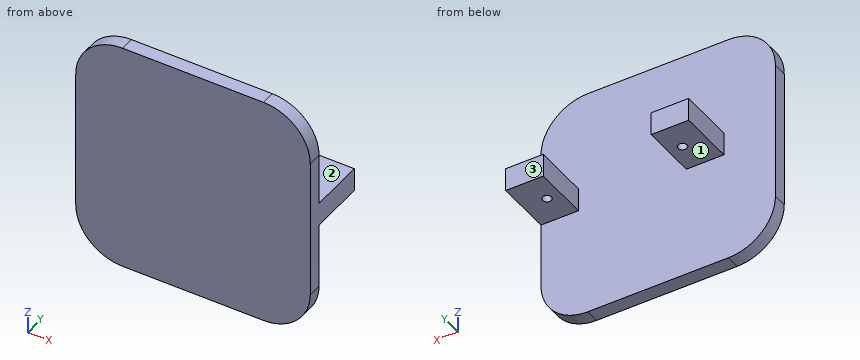
```python
from build123d import *

# Parameters (mm, degrees)
EXTRUDE_1_DEPTH     = 3
SKETCH_2_W          = 8
SKETCH_2_H          = 5
EXTRUDE_2_DEPTH     = 15
SKETCH_3_R          = 0.95
CUT_EXTRUDE_1_DEPTH = 15


with BuildPart() as part:
    # 草图1 → 凸台-拉伸1 (new body)
    with BuildSketch(Plane(origin=(0, 0, 0), x_dir=(1, 0, 0), z_dir=(0, 1, 0))):
        with BuildLine():
            Line((-15, 25), (15, 25))
            ThreePointArc((15, 25), (22.071067812, 22.071067812), (25, 15))
            Line((25, 15), (25, -15))
            ThreePointArc((25, -15), (22.071067812, -22.071067812), (15, -25))
            Line((15, -25), (-15, -25))
            ThreePointArc((-15, -25), (-22.071067812, -22.071067812), (-25, -15))
            Line((-25, -15), (-25, 15))
            ThreePointArc((-25, 15), (-22.071067812, 22.071067812), (-15, 25))
        make_face()
    extrude(amount=EXTRUDE_1_DEPTH)

    # 草图2 → 凸台-拉伸2 (add)
    with BuildSketch(Plane(origin=(0, 0, 0), x_dir=(1, 0, 0), z_dir=(0, 1, 0))):
        with Locations((21, -1.5)):
            Rectangle(SKETCH_2_W, SKETCH_2_H)
        with Locations((-10, -1.5)):
            Rectangle(SKETCH_2_W, SKETCH_2_H)
    extrude(amount=EXTRUDE_2_DEPTH)

    # 草图3 → 切除-拉伸1 (cut)
    with BuildSketch(Plane(origin=(0, 0, -1), x_dir=(-1, 0, 0), z_dir=(0, 0, -1))):
        with Locations((8.95, 9)):
            Circle(SKETCH_3_R)
        with Locations((-19.95, 9)):
            Circle(SKETCH_3_R)
    extrude(amount=-CUT_EXTRUDE_1_DEPTH, mode=Mode.SUBTRACT)


solid = part.part
```
The model under review builds one solid part; all positions refer to its coordinate system, in mm. Face numbers are marked on the shaded views. A direction names the side the tool comes from. Give positions to 0.01 mm unless a question says otherwise; leave off trailing zeros. Order: outer loops, then holes, each group sorted by start corner. A loop starts at its lowest first (then second) coordinate and runs counter-clockwise, first axis right, second up. Notation, with made-up numbers: (35.25, -28.5) - (92.25, -28.5) arc R21 ccw to (92.25, 9.5) - close; hole circle Ø7 at (46, 67). An arc over 180 degrees is marked (long way). Use CSV: the item, a comma, the result in double quotes. Start each with the question number.
Q1. Clearance check with flat-ended pins moving along their axes: pin 1 Ø5 at (x, z) = (-6.5, 16) entering from -Y; pin 2 Ø6.5 at (x, y) = (-8, 11.5) entering from -Z; pin 3 Ø1.5 at (x, z) = (-7.5, 17) entering from +Y; pin 4 Ø5.5 at (y, z) = (9, 2) entering from -X. State where each tip first meets the part, or that it passes through.
Q2. We need section B-B, the plane y = 13. Write out the cut boundary in (x, z), and give its area (3 significant figures).
Q3. Tool access review of the marked faces 1, 2 and 3: name each direction out of +Z, -Z, +X, -X, +Y, -Y from which nothing blocks a thin tool from reaching the whole face with its end or side.
Q4. We need section C-C, the plane y = 9. Write out the cut boundary in (x, z), and give its area (3 significant figures).
Q5. We need section D-D, the plane z = -21. Write out the cut boundary in (x, y), and give its area (3 significant figures).
Q6. We need section A-A, the plane x = -8.95. Write out the cut boundary in (y, z).
Q7. To check wall thickness, follow line 1 along Y through (x, z) = (19.95, 0.65); line 2 along X through (y, z) = (11, 0.5); line 3 along Z through (x, y) = (-11, 4.75). State the ranges of each line that lie inside material, in increasing order. Write a range as [from, to].
Outcome:
1,pin 1,"stops at y = 0"
1,pin 2,"stops at z = -1"
1,pin 3,"stops at y = 3"
1,pin 4,"stops at x = -14"
2,outline,"(-14, -1) - (-6, -1) - (-6, 4) - (-14, 4) - close; (17, -1) - (25, -1) - (25, 4) - (17, 4) - close"
2,area,"80.0 mm^2"
3,face 1,"-Z, +X, -X, +Y"
3,face 2,"+Z, +X, -X, +Y"
3,face 3,"+Z, -Z, +X, -X, +Y"
4,outline,"(-14, -1) - (-9.9, -1) - (-9.9, 4) - (-14, 4) - close; (-8, -1) - (-6, -1) - (-6, 4) - (-8, 4) - close; (17, -1) - (19, -1) - (19, 4) - (17, 4) - close; (20.9, -1) - (25, -1) - (25, 4) - (20.9, 4) - close"
4,area,"61.0 mm^2"
5,outline,"(-23, 0) - (23, 0) - (23, 3) - (-23, 3) - close"
5,area,"138 mm^2"
6,outline,"(0, -25) - (3, -25) - (3, -1) - (8.05, -1) - (8.05, 4) - (3, 4) - (3, 25) - (0, 25) - close; (9.95, -1) - (15, -1) - (15, 4) - (9.95, 4) - close"
7,line 1,"y = [0, 8.05], [9.95, 15]"
7,line 2,"x = [-14, -6], [17, 25]"
7,line 3,"z = [-1, 4]"
